from build123d import *

# Parameters (mm, degrees)
SKETCH_1_W          = 860
SKETCH_1_H          = 100
EXTRUDE_1_DEPTH     = 8
SKETCH_2_W          = 860
SKETCH_2_H          = 8
EXTRUDE_2_DEPTH     = 92
CUT_EXTRUDE_1_DEPTH = 453.65881191


with BuildPart() as part:
    # 草图1 → 凸台-拉伸1 (new body)
    with BuildSketch(Plane.XY):
        with Locations((0, 50)):
            Rectangle(SKETCH_1_W, SKETCH_1_H)
    extrude(amount=EXTRUDE_1_DEPTH)

    # 草图2 → 凸台-拉伸2 (add)
    with BuildSketch(Plane.XY.offset(8)):
        with Locations((0, 96)):
            Rectangle(SKETCH_2_W, SKETCH_2_H)
    extrude(amount=EXTRUDE_2_DEPTH)

    # 草图4 → 切除-拉伸1 (cut, through all)
    with BuildSketch(Plane(origin=(0, 100, 0), x_dir=(1, 0, 0), z_dir=(0, 1, 0))):
        Polygon((-430, -15), (-390, -15), (-305, -100), (-430, -100), align=None)
    cut_extrude_1 = extrude(amount=-CUT_EXTRUDE_1_DEPTH, mode=Mode.SUBTRACT)

    # 镜向1: 切除-拉伸1 across plane
    add(cut_extrude_1.mirror(Plane(origin=(0, 0, 0), x_dir=(0, 0, 1), z_dir=(1, 0, 0))), mode=Mode.SUBTRACT)


solid = part.part
Build history of the part. All positions in model axes, mm. A direction names the side the tool comes from. Coordinates: 2 decimals unless noted, no trailing zeros. Order: outer loops, then holes, each group sorted by start corner. A loop starts at its lowest first (then second) coordinate and runs counter-clockwise, first axis right, second up. Notation, with made-up numbers: M 46,-15 L 83,-15 A24 ccw 83,20 Z; hole C 35.5,71.25 d10. An arc over 180 degrees is marked long. One line per question, with ' | ' between items. Start each with the question number.
Q1. Saw through at A-A (x = -312). List the corners of the cut face in (y, z).
Q2. Probe L1, parallel to Z at x = 42, y = 51.5; L2, parallel to Y at x = 230.5, z = 69; L3, parallel to X at y = 94.5, z = 38.5. List the from-to ranges inside material, lowest first. Write a range as from..to.
Q3. Saw through at C-C (y = 63). List the corners of the cut face in (x, z).
Q4. Saw through at B-B (z = 91.5). List the corners of the cut face in (x, y).
Q5. Saw through at D-D (x = -133). List the corners of the cut face in (y, z), then the cut area to 3 significant figures.
Q6. Flat gauge pins, fed straight in: pin 1 Ø5 at (x, y) = (-203.5, 57.5) entering from +Z; pin 2 Ø6.5 at (x, y) = (-400, 95) entering from +Z; pin 3 Ø1.5 at (x, z) = (-208, 44) entering from -Y. Where does each tip first touch, or does it go through?
Q7. 3-axis set-ups, long thin cutter, end or side, ignore diameter. For faces 1 (the face through (430, 49, 4)), 2 (the face through (-6, 92, 53)): which of +Z, -Z, +X, -X, +Y, -Y reach the whole face in a straight line?
Check values:
1) outline: M 0,0 L 100,0 L 100,93 L 92,93 L 92,8 L 0,8 Z
2) L1: z = 0..8 | L2: y = 92..100 | L3: x = -366.5..366.5
3) outline: M -430,0 L 430,0 L 430,8 L -430,8 Z
4) outline: M -313.5,92 L 313.5,92 L 313.5,100 L -313.5,100 Z
5) outline: M 0,0 L 100,0 L 100,100 L 92,100 L 92,8 L 0,8 Z | area: 1,540 mm2
6) pin 1: stops at z = 8 | pin 2: stops at z = 15 | pin 3: stops at y = 92
7) face 1: +Z, -Z, +X, +Y, -Y | face 2: +Z, +X, -X, -Y
